Model file for the job. Use its own axes, mm. Face numbers are marked on the shaded views. A direction names the side the tool comes from. Give positions to 0.01 mm unless a question says otherwise; leave off trailing zeros. Order: outer loops, then holes, each group sorted by start corner. A loop starts at its lowest first (then second) coordinate and runs counter-clockwise, first axis right, second up. Notation, with made-up numbers: (75, 21) -> (107, 21) arc R8 cw to (107, 34) -> close; hole circle Ø3 at (23, -5). An arc over 180 degrees is marked (long way). Answer in a Markdown table with one row per item. Add a question column.
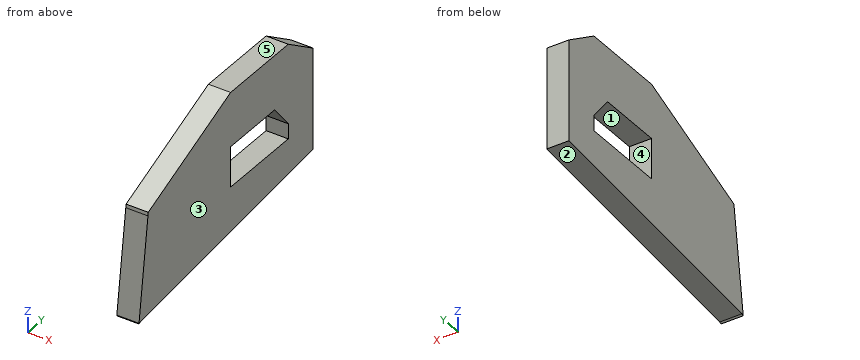
from build123d import *

# Parameters (mm, degrees)
F1_DEPTH = 25


with BuildPart() as f1:
    # F0 (on Right) → F1 (new body)
    with BuildSketch(Plane.YZ):
        Polygon((50.7914237678, 49.0828417242), (47.3742634058, 49.0828417242), (-46.7529594898, 49.0828417242), (-46.7529594898, -12.1967571052), (27.6393722743, -12.1967571052), align=None)
        Polygon((-46.7529594898, -12.1967571052), (-46.7529594898, 49.0828417242), (-186.2022727728, -8.4043648094), (-186.711434477, -12.1967571052), align=None)
        Polygon((93.0533483624, 21.0719704628), (50.7914237678, 49.0828417242), (50.7914237678, -40.7016065636), (93.0533483624, -92.734567821), align=None)
        Polygon((50.7914237678, -40.7016065636), (50.7914237678, 49.0828417242), (27.6393722743, -12.1967571052), align=None)
        Polygon((-46.7529594898, -57.7810667455), (-46.7529594898, -12.1967571052), (-186.711434477, -12.1967571052), (-201.8551233379, -124.9915892651), (-199.729913905, -124.7591343415), align=None)
        Polygon((93.0533483624, -92.734567821), (50.7914237678, -40.7016065636), (50.7914237678, -57.7810667455), align=None)
        Polygon((50.7914237678, -57.7810667455), (-46.7529594898, -57.7810667455), (-199.729913905, -124.7591343415), (93.0533483624, -92.734567821), align=None)
        Polygon((-201.9546926022, -125.7332116365), (-199.729913905, -124.7591343415), (-201.8551233379, -124.9915892651), align=None)
    extrude(amount=F1_DEPTH)


solid = f1.part
Item 1: Pin check, flat tips, straight feed: pin 1 Ø12 at (x, y) = (17, 15.5) entering from -Z; pin 2 Ø1.5 at (x, y) = (18.5, -148) entering from -Z; pin 3 Ø4 at (x, y) = (5, -65.5) entering from +Z. Stop position of each tip, or through.
Item 2: Two-plate mould, pull along Y, no slides. Class the marked faces 1, 2 and 3: pulls with the +Y half, pulls with the -Y half, needs draft (parallel to the pull), parting line crosses it, or undercut.
Item 3: Saw through at A-A on x = 21.25. List the corners of the cut face in (y, z).
Item 4: Saw through at C-C on z = 13.5. List the corners of the cut face in (x, y).
Item 5: Which spindle directions (+Z, -Z, +X, -X, +Y, -Y) get a long thin tool onto all of the face, cutting with end or side? Do the marked faces 4 and 5. Say none if no direction does.
Item 6: Saw through at B-B on y = 39.5. List the corners of the cut face in (x, z).
Item 7: Wall check: line 1 (Y direction, x = 3.75, z = -52); line 2 (Z direction, x = 12.75, y = 45.5); line 3 (Z direction, x = 18.5, y = 8). Give the ranges that are in metal, low to high.
Item 8: Saw through at D-D on y = 74. List the corners of the cut face in (x, z).
Evaluation:
| question | item | result |
|---|---|---|
| 1 | pin 1 | stops at z = -101.87 |
| 1 | pin 2 | stops at z = -119.18 |
| 1 | pin 3 | stops at z = 42.18 |
| 2 | face 1 | undercut |
| 2 | face 2 | pulls with the +Y half |
| 2 | face 3 | needs draft |
| 3 | outline | (-201.95, -125.73) -> (-199.73, -124.76) -> (93.05, -92.73) -> (93.05, 21.07) -> (50.79, 49.08) -> (-46.75, 49.08) -> (-186.2, -8.4) -> close; hole (-46.75, -57.78) -> (50.79, -57.78) -> (50.79, -40.7) -> (27.64, -12.2) -> (-46.75, -12.2) -> close |
| 4 | outline | (0, -133.07) -> (25, -133.07) -> (25, 93.05) -> (0, 93.05) -> close |
| 5 | face 4 | +X, -X |
| 5 | face 5 | +Z, +X, -X, +Y, -Y |
| 6 | outline | (0, -98.59) -> (25, -98.59) -> (25, -57.78) -> (0, -57.78) -> close; (0, -26.8) -> (25, -26.8) -> (25, 49.08) -> (0, 49.08) -> close |
| 7 | line 1 | y = -192.06 to -46.75, 50.79 to 93.05 |
| 7 | line 2 | z = -97.94 to -57.78, -34.19 to 49.08 |
| 7 | line 3 | z = -102.04 to -57.78, -12.2 to 49.08 |
| 8 | outline | (0, -94.82) -> (25, -94.82) -> (25, 33.7) -> (0, 33.7) -> close |
